Model file for the job. Use its own axes, mm. A direction names the side the tool comes from. Coordinates: 2 decimals unless noted, no trailing zeros. Write each loop counter-clockwise with the first axis right and the second up, starting at its lowest first coordinate (ties: lowest second). Pieces come first, ordered by that corner, then holes.
Q1. Band-saw the part on A-A, the plane z = 2.1. State how many separate pieces and enclosed holes the cut face has, plus the area to 3 significant figures.
Q2. Pull direction Y, two halves, no side cores. Call faces 4 (the flat face through (140, 80.45, 2)), 5 (the flat face through (142.5, 77, 2)), 6 (the cylindrical face through (131.07, 79.1, 1.73)): released by +Y, released by -Y, zero draft, split by the parting line, or undercut.
Q3. Drill centre lines: probe 1 along Y at (x, z) = (141, 3.2); probe 2 along Y at (x, z) = (146, 0.95); probe 3 along X at (y, z) = (81.75, 0.5). Where is each one in solid material? Low to high.
Q4. Band-saw the part on B-B, the plane y = 82. Write the cut outline in (x, z), plus the area to 3 significant figures.
Q5. Band-saw the part on C-C, the plane x = 143.75. Write the cut outline in (y, z), plus the area to 3 significant figures.
Q6. Pin check, flat tips, straight feed: P1, Ø0.6, axis at x = 147, z = 3, coming from the -Y side; P2, Ø1, axis at x = 139.5, z = 0.5, coming from the +Y side; P3, Ø0.6, axis at y = 80, z = 1.5, coming from the -X side. Stop position of each tip, or through.
Q7. Which spindle directions (+Z, -Z, +X, -X, +Y, -Y) get a long thin tool onto all of the face, cutting with end or side? Do faces 1 (the flat face through (140, 79.75, 2)), 2 (the flat face through (133, 78.5, 2)), 3 (the flat face through (130.5, 82, 2)). Say none if no direction does.
from build123d import *

# Parameters (mm, degrees)
SKETCH_W          = 10
SKETCH_H          = 0.7
PAD_DEPTH         = 3.5
SKETCH001_W       = 1
SKETCH001_H       = 2
POCKET_DEPTH      = 7.003756
POCKET_DEPTH_BACK = 12.007881
FILLET_R          = 1


with BuildPart() as part:
    # Sketch → Pad (new body)
    with BuildSketch(Plane.XY):
        with BuildLine():
            Line((148, 81.55), (148, 82.25))
            Line((148, 82.25), (145.25, 82.25))
            ThreePointArc((144.5, 83), (144.71967, 82.46967), (145.25, 82.25))
            ThreePointArc((145.25, 83.75), (144.71967, 83.53033), (144.5, 83))
            Line((148.75, 83.75), (145.25, 83.75))
            ThreePointArc((149.5, 83), (149.28033, 83.53033), (148.75, 83.75))
            Line((149.5, 80.5), (149.5, 83))
            ThreePointArc((147.5, 78.5), (148.914214, 79.085786), (149.5, 80.5))
            Line((146.5, 78.5), (147.5, 78.5))
            ThreePointArc((146.5, 78.5), (145.085786, 77.914214), (144.5, 76.5))
            Line((144.5, 76.395912), (144.5, 76.5))
            Line((142.5, 76.395912), (144.5, 76.395912))
            Line((142.5, 76.395912), (142.5, 78.5))
            Line((142.5, 78.5), (137.5, 78.5))
            Line((137.5, 78.5), (137.502762, 76.395912))
            Line((135.502762, 76.395912), (137.502762, 76.395912))
            Line((135.5, 76.5), (135.502762, 76.395912))
            ThreePointArc((135.5, 76.5), (134.914214, 77.914214), (133.5, 78.5))
            Line((133.5, 78.5), (132.5, 78.5))
            ThreePointArc((130.5, 80.5), (131.085786, 79.085786), (132.5, 78.5))
            Line((130.5, 83), (130.5, 80.5))
            ThreePointArc((131.25, 83.75), (130.71967, 83.53033), (130.5, 83))
            Line((131.25, 83.75), (134.75, 83.75))
            ThreePointArc((135.5, 83), (135.28033, 83.53033), (134.75, 83.75))
            ThreePointArc((134.75, 82.25), (135.28033, 82.46967), (135.5, 83))
            Line((132, 82.25), (134.75, 82.25))
            Line((132, 82.25), (132, 81.55))
            Line((132, 81.55), (148, 81.55))
        make_face()
        with Locations((140, 80.1)):
            Rectangle(SKETCH_W, SKETCH_H, mode=Mode.SUBTRACT)
    extrude(amount=PAD_DEPTH)

    # Sketch001 (on DatumPlane) → Pocket (cut, two sides)
    with BuildSketch(Plane(origin=(137.602808, 0.180629, 0), x_dir=(-0.001313, 0.999999, 0), z_dir=(0.999999, 0.001313, 0))) as pocket_sk:
        with Locations((77.819439, 1.76189)):
            Rectangle(SKETCH001_W, SKETCH001_H)
    extrude(amount=-POCKET_DEPTH, mode=Mode.SUBTRACT)
    extrude(pocket_sk.sketch, amount=POCKET_DEPTH_BACK, mode=Mode.SUBTRACT)

    # Fillet
    fillet_edges = [part.edges().sort_by_distance(p)[0] for p in [
        (143.5, 76.395912, 3.5),
        (136.502762, 76.395912, 3.5),
    ]]
    fillet(fillet_edges, radius=FILLET_R)


solid = part.part
Answer sheet:
1. separate pieces: 3
1. enclosed holes: 1
1. area: 70.2 mm2
2. face 4: undercut
2. face 5: zero draft
2. face 6: released by -Y
3. probe 1: y = 78.5 to 79.75, 80.45 to 81.55
3. probe 2: y = 78.51 to 81.55, 82.25 to 83.75
3. probe 3: x = 130.5 to 132, 148 to 149.5
4. outline: (130.5, 0) - (132, 0) - (132, 3.5) - (130.5, 3.5) - close; (148, 0) - (149.5, 0) - (149.5, 3.5) - (148, 3.5) - close
4. area: 10.5 mm2
5. outline: (76.4, 0) - (79.75, 0) - (79.75, 3.5) - (77.4, 3.5) arc R1 ccw to (76.4, 2.5) - close; (80.45, 0) - (81.55, 0) - (81.55, 3.5) - (80.45, 3.5) - close; hole (77.51, 0.76) - (78.51, 0.76) - (78.51, 2.76) - (77.51, 2.76) - close
5. area: 13.4 mm2
6. P1: stops at y = 78.5
6. P2: stops at y = 81.55
6. P3: stops at x = 130.51
7. face 1: +Z, -Z
7. face 2: +Z, -Z, -X, -Y
7. face 3: +Z, -Z, -X, +Y, -Y
